from build123d import *

# Parameters (mm, degrees)
ESQUISSE1_W             = 5
ESQUISSE1_H             = 5
BOSS_EXTRU_1_DEPTH      = 10
ESQUISSE2_R             = 1.5
ENL_V_MAT_EXTRU_1_DEPTH = 13.247448714


with BuildPart() as part:
    # Esquisse1 → Boss.-Extru.1 (new body)
    with BuildSketch(Plane.XY):
        with Locations((2.5, 2.5)):
            Rectangle(ESQUISSE1_W, ESQUISSE1_H)
    extrude(amount=BOSS_EXTRU_1_DEPTH)

    # Esquisse2 → Enlèv. mat.-Extru.1 (cut, through all)
    with BuildSketch(Plane.XY.offset(10)):
        with Locations((2.5, 2.5)):
            Circle(ESQUISSE2_R)
        with BuildLine():
            ThreePointArc((5, 2.5), (4.267766953, 0.732233047), (2.5, 0))
            Line((2.5, 0), (5, 0))
            Line((5, 0), (5, 2.5))
        make_face()
        with BuildLine():
            ThreePointArc((2.5, 0), (0.732233047, 0.732233047), (0, 2.5))
            Line((0, 2.5), (0, 0))
            Line((0, 0), (2.5, 0))
        make_face()
    extrude(amount=-ENL_V_MAT_EXTRU_1_DEPTH, mode=Mode.SUBTRACT)


solid = part.part
The model under review builds one solid part; all positions refer to its coordinate system, in mm. Give positions to 0.01 mm unless a question says otherwise; leave off trailing zeros. Loops run counter-clockwise (first coordinate to the right, second up) from the corner with the lowest first, then second, coordinate; pieces in that order, holes last. Notation, with made-up numbers: (59.25, -33.75) -> (73.25, -33.75) arc R14 ccw to (73.25, -18.75) -> close; hole circle Ø5 at (40.5, 57.5). An arc over 180 degrees is marked (long way). Put each result on its own line as item: value. Start each with the question number.
1. Clearance check with flat-ended pins moving along their axes: P1, Ø1, axis at y = 2.5, z = 3.5, coming from the -X side; P2, Ø2, axis at x = 4, z = 6.5, coming from the -Y side. State where each tip first meets the part, or that it passes through.
2. We need section C-C on z = 4. State the section outline as (x, y) points, then the cut area to 3 significant figures.
3. We need section B-B on x = 3.45. State the section outline as (y, z) points.
4. Mouldability with a two-part tool opening along X and no side actions: class faces 1 (the face through (5, 4, 5)), 2 (the face through (4, 4, 0)), 3 (the face through (2.175, 1.036, 5.07)) as released by +X, released by -X, zero draft, split by the parting line, or undercut.
5. We need section A-A on y = 2.8. State the section outline as (x, z) points, then the cut area to 3 significant figures.
6. Wall thickness on probe 1 along Y at (x, z) = (2.5, 3.75); probe 2 along X at (y, z) = (3.3, 1.75); probe 3 along X at (y, z) = (3.35, 5.25): over which ranges is each line inside the solid? List them lowest first.
Determined:
1. P1: x = 0
1. P2: y = 0.05
2. outline: (0, 2.5) arc R2.5 ccw to (5, 2.5) -> (5, 5) -> (0, 5) -> close; hole circle Ø3 at (2.5, 2.5)
2. area: 15.2 mm^2
3. outline: (0.19, 0) -> (1.34, 0) -> (1.34, 10) -> (0.19, 10) -> close; (3.66, 0) -> (5, 0) -> (5, 10) -> (3.66, 10) -> close
4. face 1: released by +X
4. face 2: zero draft
4. face 3: undercut
5. outline: (0, 0) -> (1.03, 0) -> (1.03, 10) -> (0, 10) -> close; (3.97, 0) -> (5, 0) -> (5, 10) -> (3.97, 10) -> close
5. area: 20.6 mm^2
6. probe 1: 0 to 1, 4 to 5
6. probe 2: 0 to 1.23, 3.77 to 5
6. probe 3: 0 to 1.26, 3.74 to 5
